Design review of the part built by this model. Coordinates are the model's own, in mm. Face numbers are marked on the shaded views. A direction names the side the tool comes from. Round coordinates to 2 decimals unless told otherwise and drop trailing zeros. Write each loop counter-clockwise with the first axis right and the second up, starting at its lowest first coordinate (ties: lowest second). Pieces come first, ordered by that corner, then holes. Notation, with made-up numbers: M 69.5,87 L 86.5,87 A22 ccw 86.5,96 Z; hole C 67,-2.75 d6. An arc over 180 degrees is marked long. One line per question, with ' | ' between items. Start each with the question number.
Item 1: Add section A-A, the plane y = -2. State the section outline as (x, z) points, and give its area (3 significant figures).
Item 2: Insertion check: pin 1 Ø0.6 at (y, z) = (-9, 11.5) entering from +X; pin 2 Ø5 at (x, z) = (-59.5, -19.5) entering from -Y; pin 3 Ø3.5 at (x, z) = (21.5, 41.5) entering from +Y; pin 4 Ø2.5 at (x, z) = (11.25, 0) entering from -Y. Each pin has a flat end and moves straight along its axis. Give the tip position at first contact, or say it passes through.
Item 3: Add section B-B, the plane x = -33.75. State the section outline as (y, z) points.
Item 4: Add section D-D, the plane x = -53. State the section outline as (y, z) points.
Item 5: Machinability: for the marked faces 4, 5 and 6, which of the approach directions +Z, -Z, +X, -X, +Y, -Y give a long, thin tool a straight path to every point of the face, cutting with its end or side? Answer none if there is none.
Item 6: Draft analysis for pull direction Z (two halves, no side actions). For the marked faces 1, 2 and 3, state which applies: released by +Z, released by -Z, zero draft, split by the parting line, or undercut.
Item 7: For L1, parallel to X at y = 10.5, z = 14; L2, parallel to X at y = 2, z = -10; L3, parallel to Z at x = -6, y = -2.5, list the stretches that pass through material, from the lowest coordinate up.
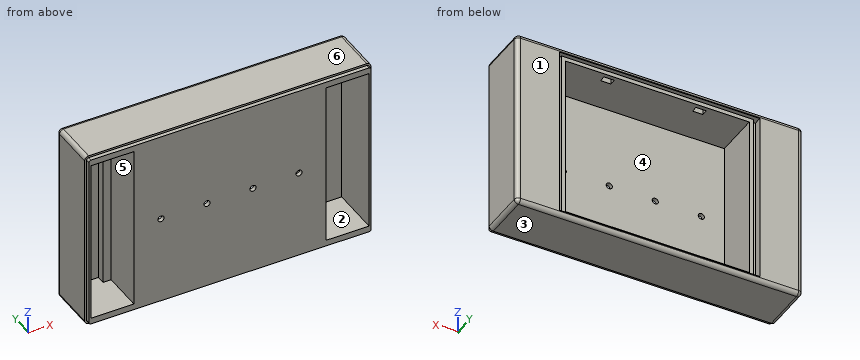
```python
from build123d import *

# Parameters (mm, degrees)
BOSS_EXTRUDE1_DEPTH      = 16
BOSS_EXTRUDE1_DEPTH_BACK = 10
SKETCH1_W                = 140
SKETCH1_H                = 89
SKETCH2_W                = 94
SKETCH2_H                = 84
BOSS_EXTRUDE2_DEPTH      = 22
SKETCH3_W                = 90
SKETCH3_H                = 80
CUT_EXTRUDE2_DEPTH       = 24
SKETCH5_R                = 1.5
CUT_EXTRUDE4_DEPTH       = 2
FILLET1_R                = 2
FILLET2_R                = 2
CUT_EXTRUDE8_DEPTH       = 2
SKETCH10_W               = 5
SKETCH10_H               = 3
CUT_EXTRUDE9_DEPTH       = 3
SKETCH11_W               = 2
SKETCH11_H               = 84
CUT_EXTRUDE10_DEPTH      = 2
SHELL1_START             = -68
SHELL1_OUTLINE_W         = 20
SHELL1_OUTLINE_H         = 81
SHELL1_DEPTH             = 21
SHELL1_START_2           = 47
SHELL1_2_OUTLINE_W       = 20
SHELL1_2_OUTLINE_H       = 81
SHELL1_2_DEPTH           = 21
SHELL1_3_OUTLINE_W       = 4
SHELL1_3_OUTLINE_H       = 81
SHELL1_3_DEPTH           = 17
SHELL1_START_3           = 51
SHELL1_4_OUTLINE_W       = 4
SHELL1_4_OUTLINE_H       = 81
SHELL1_4_DEPTH           = 17
SKETCH7_OUTSIDE_W        = 175.584
SKETCH7_OUTSIDE_H        = 124.584
CUT_EXTRUDE6_DEPTH       = 2


# Read off the part's stored shape, not the designer's step: Shell1
with BuildPart() as part:
    # Sketch1 → Boss-Extrude1 (new, two sides: drawn at the far end of the back side and taken through both)
    with BuildSketch(Plane(origin=(0, 0, 0), x_dir=(1, 0, 0), z_dir=(0, 1, 0)).offset(-BOSS_EXTRUDE1_DEPTH_BACK)):
        Rectangle(SKETCH1_W, SKETCH1_H)
    extrude(amount=BOSS_EXTRUDE1_DEPTH + BOSS_EXTRUDE1_DEPTH_BACK)

    # Sketch2 → Boss-Extrude2 (add)
    with BuildSketch(Plane(origin=(0, 16, 0), x_dir=(1, 0, 0), z_dir=(0, 1, 0))):
        Rectangle(SKETCH2_W, SKETCH2_H)
    extrude(amount=-BOSS_EXTRUDE2_DEPTH)

    # Sketch3 → Cut-Extrude2 (cut)
    with BuildSketch(Plane(origin=(0, 16, 0), x_dir=(1, 0, 0), z_dir=(0, 1, 0))):
        Rectangle(SKETCH3_W, SKETCH3_H)
    extrude(amount=-CUT_EXTRUDE2_DEPTH, mode=Mode.SUBTRACT)

    # Sketch5 → Cut-Extrude4 (cut)
    with BuildSketch(Plane(origin=(0, -8, 0), x_dir=(1, 0, 0), z_dir=(0, 1, 0))):
        with Locations(Location((-33.75, 0, 0), (0, 0, 270))):
            Circle(SKETCH5_R)
        with Locations(Location((-11.25, 0, 0), (0, 0, 270))):
            Circle(SKETCH5_R)
        with Locations(Location((11.25, 0, 0), (0, 0, 270))):
            Circle(SKETCH5_R)
        with Locations(Location((33.75, 0, 0), (0, 0, 270))):
            Circle(SKETCH5_R)
    extrude(amount=-CUT_EXTRUDE4_DEPTH, mode=Mode.SUBTRACT)

    # Fillet1
    fillet1_edges = [part.edges().sort_by_distance(p)[0] for p in [
        (70, 3, 44.5),
        (-70, 3, 44.5),
        (-70, 3, -44.5),
        (70, 3, -44.5),
    ]]
    fillet(fillet1_edges, radius=FILLET1_R)

    # Fillet2
    fillet2_edges = [part.edges().sort_by_distance(p)[0] for p in [
        (-70, 16, 0),
        (70, 16, 0),
        (0, 16, -44.5),
        (0, 16, 44.5),
        (69.414213562, 16, 43.914213562),
        (69.414213562, 16, -43.914213562),
        (-69.414213562, 16, -43.914213562),
        (-69.414213562, 16, 43.914213562),
    ]]
    fillet(fillet2_edges, radius=FILLET2_R)

    # Sketch8 → Cut-Extrude8 (cut)
    with BuildSketch(Plane(origin=(0, 16, 0), x_dir=(1, 0, 0), z_dir=(0, 1, 0))):
        Polygon((-47, 42), (-49, 42), (-49, -42), (-47, -42), (47, -42), (49, -42), (49, 42), (47, 42), align=None)
    extrude(amount=-CUT_EXTRUDE8_DEPTH, mode=Mode.SUBTRACT)

    # Sketch10 → Cut-Extrude9 (cut)
    with BuildSketch(Plane(origin=(0, 0, 40), x_dir=(-1, 0, 0), z_dir=(0, 0, -1))):
        with Locations((-22.5, 10.5)):
            Rectangle(SKETCH10_W, SKETCH10_H)
        with Locations((22.5, 10.5)):
            Rectangle(SKETCH10_W, SKETCH10_H)
    extrude(amount=-CUT_EXTRUDE9_DEPTH, mode=Mode.SUBTRACT)

    # Sketch11 → Cut-Extrude10 (cut)
    with BuildSketch(Plane(origin=(0, 14, 0), x_dir=(1, 0, 0), z_dir=(0, 1, 0))):
        with Locations((-48, 0)):
            Rectangle(SKETCH11_W, SKETCH11_H)
        with Locations((48, 0)):
            Rectangle(SKETCH11_W, SKETCH11_H)
    extrude(amount=-CUT_EXTRUDE10_DEPTH, mode=Mode.SUBTRACT)

    # Shell1 outline → Shell1 (cut)
    with BuildSketch(Plane.YZ.offset(SHELL1_START)):
        Rectangle(SHELL1_OUTLINE_W, SHELL1_OUTLINE_H)
    extrude(amount=SHELL1_DEPTH, mode=Mode.SUBTRACT)

    # Shell1 2 outline → Shell1 2 (cut)
    with BuildSketch(Plane.YZ.offset(SHELL1_START_2)):
        Rectangle(SHELL1_2_OUTLINE_W, SHELL1_2_OUTLINE_H)
    extrude(amount=SHELL1_2_DEPTH, mode=Mode.SUBTRACT)

    # Shell1 3 outline → Shell1 3 (cut)
    with BuildSketch(Plane.YZ.offset(SHELL1_START)):
        with Locations((12, 0)):
            Rectangle(SHELL1_3_OUTLINE_W, SHELL1_3_OUTLINE_H)
    extrude(amount=SHELL1_3_DEPTH, mode=Mode.SUBTRACT)

    # Shell1 4 outline → Shell1 4 (cut)
    with BuildSketch(Plane.YZ.offset(SHELL1_START_3)):
        with Locations((12, 0)):
            Rectangle(SHELL1_4_OUTLINE_W, SHELL1_4_OUTLINE_H)
    extrude(amount=SHELL1_4_DEPTH, mode=Mode.SUBTRACT)

    # Sketch7 outside → Cut-Extrude6 (cut)
    with BuildSketch(Plane.XZ.offset(10)):
        Rectangle(SKETCH7_OUTSIDE_W, SKETCH7_OUTSIDE_H)
        with BuildLine():
            Line((-68, -43.5), (68, -43.5))
            ThreePointArc((68, -43.5), (68.707106781, -43.207106781), (69, -42.5))
            Line((69, -42.5), (69, 42.5))
            ThreePointArc((69, 42.5), (68.707106781, 43.207106781), (68, 43.5))
            Line((68, 43.5), (-68, 43.5))
            ThreePointArc((-68, 43.5), (-68.707106781, 43.207106781), (-69, 42.5))
            Line((-69, 42.5), (-69, -42.5))
            ThreePointArc((-69, -42.5), (-68.707106781, -43.207106781), (-68, -43.5))
        make_face(mode=Mode.SUBTRACT)
    extrude(amount=-CUT_EXTRUDE6_DEPTH, mode=Mode.SUBTRACT)


solid = part.part
```
Computed values:
1) outline: M -70,-42.5 A2 ccw -68,-44.5 L 68,-44.5 A2 ccw 70,-42.5 L 70,42.5 A2 ccw 68,44.5 L -68,44.5 A2 ccw -70,42.5 Z; hole M -68,-40.5 L -47,-40.5 L -47,40.5 L -68,40.5 Z; hole M -45,-40 L 45,-40 L 45,40 L -45,40 Z; hole M 47,-40.5 L 68,-40.5 L 68,40.5 L 47,40.5 Z | area: 1,850 mm^2
2) pin 1: stops at x = 69 | pin 2: stops at y = 14 | pin 3: stops at y = 16 | pin 4: passes through
3) outline: M -10,-43.5 L -8,-43.5 L -8,-44.5 L 14,-44.5 A2 ccw 16,-42.5 L 16,-42 L 14,-42 L 14,-40 L -8,-40 L -8,-1.5 L -10,-1.5 Z; M -10,1.5 L -8,1.5 L -8,40 L 14,40 L 14,42 L 16,42 L 16,42.5 A2 ccw 14,44.5 L -8,44.5 L -8,43.5 L -10,43.5 Z
4) outline: M -10,-43.5 L -8,-43.5 L -8,-44.5 L 14,-44.5 A2 ccw 16,-42.5 L 16,42.5 A2 ccw 14,44.5 L -8,44.5 L -8,43.5 L -10,43.5 L -10,40.5 L 14,40.5 L 14,-40.5 L -10,-40.5 Z
5) face 4: +Y | face 5: -Y | face 6: +Z, +X, -X, +Y, -Y
6) face 1: zero draft | face 2: undercut | face 3: released by -Z
7) L1: x = -70 to -68, -51 to -45, 45 to 51, 68 to 70 | L2: x = -70 to -68, -47 to -45, 45 to 47, 68 to 70 | L3: z = -44.5 to -40, 40 to 44.5
